For this review, take the finished solid that the model builds, in its own axes (mm). Face numbers are marked on the shaded views. A direction names the side the tool comes from. Coordinates: 2 decimals unless noted, no trailing zeros. Order: outer loops, then holes, each group sorted by start corner. A loop starts at its lowest first (then second) coordinate and runs counter-clockwise, first axis right, second up. Notation, with made-up numbers: (1, 21) -> (17, 21) arc R30 cw to (17, 52) -> close; hole circle Ø3 at (70, -9.75). An arc over 180 degrees is marked (long way). Answer as a JSON object with one key per item and string values. Group by question number.
1) Add section A-A, the plane y = 14.25. Write out the cut boundary in (x, z), then the cut area to 3 significant figures.
2) Machinability: for the marked faces 1 and 2, which of the approach directions +Z, -Z, +X, -X, +Y, -Y give a long, thin tool a straight path to every point of the face, cutting with its end or side? Answer none if there is none.
3) Add section D-D, the plane z = 8.5. Write out the cut boundary in (x, y).
4) For pin 1 (12 mm diameter, centred on x = 6.5, y = 13.5, fed in from +Z); pin 2 (1.5 mm diameter, centred on y = 19.5, z = 8.5, fed in from +X), all flat-tipped, find the tip position at first contact; note any pin that passes through.
5) Add section B-B, the plane z = 5. Write out the cut boundary in (x, y).
6) Wall thickness on L1, parallel to X at y = 0.4, z = 5; L2, parallel to Y at x = 23, z = 6.5: over which ranges is each line inside the solid? List them lowest first.
7) Add section C-C, the plane x = 7. Write out the cut boundary in (y, z).
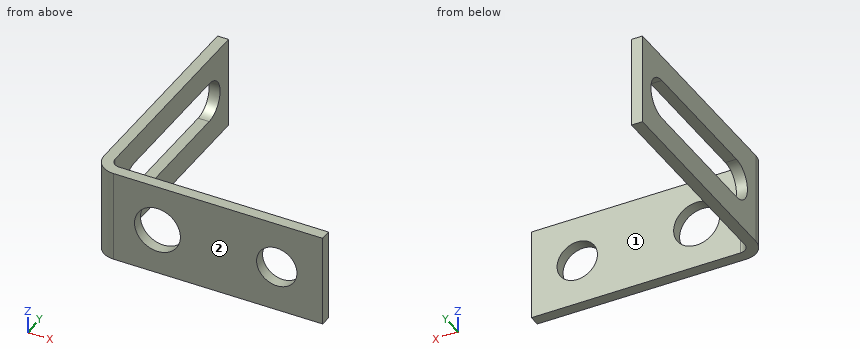
from build123d import *

# Parameters (mm, degrees)
T_LE_DE_BASE_PLI_E1_DEPTH = 10
ENL_V_MAT_EXTRU_1_REACH   = 37.937
ESQUISSE6_R               = 2.2
ESQUISSE6_R_2             = 2.5
ENL_V_MAT_EXTRU_2_REACH   = 37.937


# Sheet-metal steps are written as plain solids
with BuildPart() as part:
    # Esquisse1 → Tôle de base pliée1 (new body)
    with BuildSketch(Plane.XY):
        with BuildLine():
            Line((0, 25), (0, 2.2))
            ThreePointArc((0, 2.2), (0.644365081, 0.644365081), (2.2, 0))
            Line((2.2, 0), (25, 0))
            Line((25, 0), (25, 1.2))
            Line((25, 1.2), (2.2, 1.2))
            ThreePointArc((2.2, 1.2), (1.492893219, 1.492893219), (1.2, 2.2))
            Line((1.2, 2.2), (1.2, 25))
            Line((1.2, 25), (0, 25))
        make_face()
    extrude(amount=T_LE_DE_BASE_PLI_E1_DEPTH)

    # Esquisse6 → Enlèv. mat.-Extru.1 (cut, up to next)
    with BuildSketch(Plane(origin=(0, 1.2, 0), x_dir=(1, 0, 0), z_dir=(0, 1, 0)), mode=Mode.PRIVATE) as enl_v_mat_extru_1_sk1:
        with Locations(Location((20, -5, 0), (0, 0, 270))):
            Circle(ESQUISSE6_R)
    enl_v_mat_extru_1_tool1 = extrude(enl_v_mat_extru_1_sk1.sketch, amount=-ENL_V_MAT_EXTRU_1_REACH, mode=Mode.PRIVATE) & part.part
    # Esquisse6 → Enlèv. mat.-Extru.1 (cut, up to next)
    with BuildSketch(Plane(origin=(0, 1.2, 0), x_dir=(1, 0, 0), z_dir=(0, 1, 0)), mode=Mode.PRIVATE) as enl_v_mat_extru_1_sk2:
        with Locations(Location((7, -5, 0), (0, 0, 270))):
            Circle(ESQUISSE6_R_2)
    enl_v_mat_extru_1_tool2 = extrude(enl_v_mat_extru_1_sk2.sketch, amount=-ENL_V_MAT_EXTRU_1_REACH, mode=Mode.PRIVATE) & part.part
    add(enl_v_mat_extru_1_tool1.solids().sort_by_distance((20, 1.2, 5))[0], mode=Mode.SUBTRACT)
    add(enl_v_mat_extru_1_tool2.solids().sort_by_distance((7, 1.2, 5))[0], mode=Mode.SUBTRACT)

    # Esquisse7 → Enlèv. mat.-Extru.2 (cut, up to next)
    with BuildSketch(Plane(origin=(1.2, 0, 0), x_dir=(0, 0, -1), z_dir=(1, 0, 0)), mode=Mode.PRIVATE) as enl_v_mat_extru_2_sk1:
        with BuildLine():
            Line((-2.8, 21.1), (-2.8, 6.1))
            ThreePointArc((-2.8, 6.1), (-5, 3.9), (-7.2, 6.1))
            Line((-7.2, 6.1), (-7.2, 21.1))
            ThreePointArc((-7.2, 21.1), (-5, 23.3), (-2.8, 21.1))
        make_face()
    enl_v_mat_extru_2_tool1 = extrude(enl_v_mat_extru_2_sk1.sketch, amount=-ENL_V_MAT_EXTRU_2_REACH, mode=Mode.PRIVATE) & part.part
    add(enl_v_mat_extru_2_tool1.solids().sort_by_distance((1.2, 13.6, 5))[0], mode=Mode.SUBTRACT)


solid = part.part
Output values:
{
 "1": {"outline": "(0, 0) -> (1.2, 0) -> (1.2, 2.8) -> (0, 2.8) -> close; (0, 7.2) -> (1.2, 7.2) -> (1.2, 10) -> (0, 10) -> close", "area": "6.72 mm²"},
 "2": {"face 1": "+Z, -Z, +X, +Y", "face 2": "+Z, -Z, +X, -X, -Y"},
 "3": {"outline": "(0, 2.2) arc R2.2 ccw to (2.2, 0) -> (25, 0) -> (25, 1.2) -> (2.2, 1.2) arc R1 cw to (1.2, 2.2) -> (1.2, 25) -> (0, 25) -> close"},
 "4": {"pin 1": "stops at z = 10", "pin 2": "stops at x = 1.2"},
 "5": {"outline": "(0, 2.2) arc R2.2 ccw to (2.2, 0) -> (4.5, 0) -> (4.5, 1.2) -> (2.2, 1.2) arc R1 cw to (1.2, 2.2) -> (1.2, 3.9) -> (0, 3.9) -> close; (0, 23.3) -> (1.2, 23.3) -> (1.2, 25) -> (0, 25) -> close; (9.5, 0) -> (17.8, 0) -> (17.8, 1.2) -> (9.5, 1.2) -> close; (22.2, 0) -> (25, 0) -> (25, 1.2) -> (22.2, 1.2) -> close"},
 "6": {"L1": "x = 0.94 to 4.5, 9.5 to 17.8, 22.2 to 25", "L2": "y = 0 to 1.2"},
 "7": {"outline": "(0, 0) -> (1.2, 0) -> (1.2, 2.5) -> (0, 2.5) -> close; (0, 7.5) -> (1.2, 7.5) -> (1.2, 10) -> (0, 10) -> close"}
}
